```python
from build123d import *

# Parameters (mm, degrees)
F0_W          = 106.6800057888
F0_H          = 76.8927261233
F1_DEPTH      = 59.436
F2_W          = 84.9745497108
F2_H          = 58.4200024605
F3_DEPTH      = 59.437
F5_DEPTH      = 80.772
F5_DEPTH_BACK = 74.422
F6_R          = 7.5638145865
F7_DEPTH      = 66.548
F7_DEPTH_BACK = 73.152


with BuildPart() as f1:
    # F0 (on Top) → F1 (new body)
    with BuildSketch(Plane.XY):
        Rectangle(F0_W, F0_H)
    extrude(amount=F1_DEPTH)

    # F2 (on Top) → F3 (cut, through all)
    with BuildSketch(Plane.XY):
        Rectangle(F2_W, F2_H)
    extrude(amount=F3_DEPTH, mode=Mode.SUBTRACT)

    # F4 (on Front) → F5 (cut, two sides)
    with BuildSketch(Plane.XZ) as f5_sk:
        Polygon((34.867271781, 64.3081814051), (-33.7127298117, 64.0772730112), (-33.7127298117, 22.2827270627), (35.0981801748, 22.2827270627), align=None)
    extrude(amount=F5_DEPTH, mode=Mode.SUBTRACT)
    extrude(f5_sk.sketch, amount=-F5_DEPTH_BACK, mode=Mode.SUBTRACT)

    # F6 (on Right) → F7 (cut, two sides)
    with BuildSketch(Plane.YZ) as f7_sk:
        with Locations((0, 34.751817584)):
            Circle(F6_R)
    extrude(amount=-F7_DEPTH, mode=Mode.SUBTRACT)
    extrude(f7_sk.sketch, amount=F7_DEPTH_BACK, mode=Mode.SUBTRACT)


solid = f1.part
```
Model file for the job. Use its own axes, mm. A direction names the side the tool comes from. Coordinates: 2 decimals unless noted, no trailing zeros. Order: outer loops, then holes, each group sorted by start corner. A loop starts at its lowest first (then second) coordinate and runs counter-clockwise, first axis right, second up. Notation, with made-up numbers: (82, 24) -> (96, 24) arc R19 ccw to (96, 42) -> close; hole circle Ø11 at (0, 59). An arc over 180 degrees is marked (long way). Answer as a JSON object with one key per item and string values. Group by question number.
1) Flat gauge pins, fed straight in: pin 1 (3 mm diameter, centred on x = -6, y = 35.5, fed in from +Z); pin 2 (12 mm diameter, centred on y = 0, z = 34.75, fed in from -X). Where does each tip first touch, or does it go through?
2) Cut at B-B, the plane z = 16.5. Write the cut outline in (x, y).
3) Cut at D-D, the plane z = 31.5. Write the cut outline in (x, y), then the cut area to 3 significant figures.
4) Pull direction Z, two halves, no side cores. Call faces 4 (the face through (53.34, -1, 23)), 5 (the face through (-46, 1, 59.436)), 6 (the face through (47.838, -1.64, 27.368)): +Z half, -Z half, draft (parallel to the pull), parting line (faces both ways), or undercut.
5) Drill centre lines: L1, parallel to X at y = -29, z = 48; L2, parallel to Y at x = -30, z = 16.5; L3, parallel to Z at x = 48, y = 0. Where is each one in solid material? Low to high.
6) Which spindle directions (+Z, -Z, +X, -X, +Y, -Y) get a long thin tool onto all of the face, cutting with end or side? Do faces 1 (the face through (-1, -34, 0)), 2 (the face through (-33.713, -34, 41)), 3 (the face through (-1, -29.21, 16)). Say none if no direction does.
7) Cut at A-A, the plane x = 14.5. Write the cut outline in (y, z).
8) Cut at C-C, the plane y = 0. Write the cut outline in (x, z).
Check values:
{
 "1": {"pin 1": "stops at z = 22.28", "pin 2": "passes through"},
 "2": {"outline": "(-53.34, -38.45) -> (53.34, -38.45) -> (53.34, 38.45) -> (-53.34, 38.45) -> close; hole (-42.49, -29.21) -> (42.49, -29.21) -> (42.49, 29.21) -> (-42.49, 29.21) -> close"},
 "3": {"outline": "(-53.34, -38.45) -> (-33.71, -38.45) -> (-33.71, -29.21) -> (-42.49, -29.21) -> (-42.49, -6.83) -> (-53.34, -6.83) -> close; (-53.34, 6.83) -> (-42.49, 6.83) -> (-42.49, 29.21) -> (-33.71, 29.21) -> (-33.71, 38.45) -> (-53.34, 38.45) -> close; (35.05, -38.45) -> (53.34, -38.45) -> (53.34, -6.83) -> (42.49, -6.83) -> (42.49, -29.21) -> (35.05, -29.21) -> close; (35.05, 29.21) -> (42.49, 29.21) -> (42.49, 6.83) -> (53.34, 6.83) -> (53.34, 38.45) -> (35.05, 38.45) -> close", "area": "1,670 mm²"},
 "4": {"face 4": "draft", "face 5": "+Z half", "face 6": "undercut"},
 "5": {"L1": "x = -53.34 to -42.49, 42.49 to 53.34", "L2": "y = -38.45 to -29.21, 29.21 to 38.45", "L3": "z = 0 to 27.19, 42.32 to 59.44"},
 "6": {"face 1": "-Z, +X, -X, +Y, -Y", "face 2": "+Z, +Y, -Y", "face 3": "+Z, -Z"},
 "7": {"outline": "(-38.45, 0) -> (-29.21, 0) -> (-29.21, 22.28) -> (-38.45, 22.28) -> close; (29.21, 0) -> (38.45, 0) -> (38.45, 22.28) -> (29.21, 22.28) -> close"},
 "8": {"outline": "(-53.34, 0) -> (-42.49, 0) -> (-42.49, 27.19) -> (-53.34, 27.19) -> close; (-53.34, 42.32) -> (-42.49, 42.32) -> (-42.49, 59.44) -> (-53.34, 59.44) -> close; (42.49, 0) -> (53.34, 0) -> (53.34, 27.19) -> (42.49, 27.19) -> close; (42.49, 42.32) -> (53.34, 42.32) -> (53.34, 59.44) -> (42.49, 59.44) -> close"}
}
